Could you check a few things on this model? Use its own coordinates, in mm. Face numbers are marked on the shaded views. A direction names the side the tool comes from. Give positions to 0.01 mm unless a question says otherwise; leave off trailing zeros. Order: outer loops, then holes, each group sorted by start corner. A loop starts at its lowest first (then second) coordinate and runs counter-clockwise, first axis right, second up. Notation, with made-up numbers: (-25.75, -35) -> (-5.75, -35) arc R9 cw to (-5.75, -29) -> close; hole circle Ø7 at (21, 38.5). An arc over 180 degrees is marked (long way). Use one line per item in the form item = value. Start each with the question number.
from build123d import *

# Parameters (mm, degrees)
BOSS_EXTRUDE1_DEPTH = 4
CHAMFER1_SIZE       = 2


with BuildPart() as part:
    # Sketch2 → Boss-Extrude1 (new body)
    with BuildSketch(Plane(origin=(0, 0, 0), x_dir=(1, 0, 0), z_dir=(0, 1, 0))):
        Polygon((18, 8.5), (22.5, 8.5), (22.5, -8.5), (18, -8.5), (18, -13.5), (-18, -13.5), (-18, -8.5), (-22.5, -8.5), (-22.5, 8.5), (-18, 8.5), (-18, 13.5), (18, 13.5), align=None)
        Polygon((-8.5, -8.5), (8.5, -8.5), (0, -3), align=None, mode=Mode.SUBTRACT)
        Polygon((-4, 0), (-13, 6.5), (-13, 3.5), (-18, 3.5), (-18, -3.5), (-13, -3.5), (-13, -6.5), align=None, mode=Mode.SUBTRACT)
        Polygon((-8.5, 8.5), (0, 3), (8.5, 8.5), align=None, mode=Mode.SUBTRACT)
        Polygon((4, 0), (13, -6.5), (13, -3.5), (18, -3.5), (18, 3.5), (13, 3.5), (13, 6.5), align=None, mode=Mode.SUBTRACT)
    extrude(amount=BOSS_EXTRUDE1_DEPTH)

    # Chamfer1
    chamfer1_edges = [part.edges().sort_by_distance(p)[0] for p in [
        (22.5, 2, -8.5),
        (22.5, 2, 8.5),
        (18, 2, 13.5),
        (-18, 2, 13.5),
        (-22.5, 2, 8.5),
        (-22.5, 2, -8.5),
        (-18, 2, -13.5),
        (18, 2, -13.5),
    ]]
    chamfer(chamfer1_edges, length=CHAMFER1_SIZE)


solid = part.part
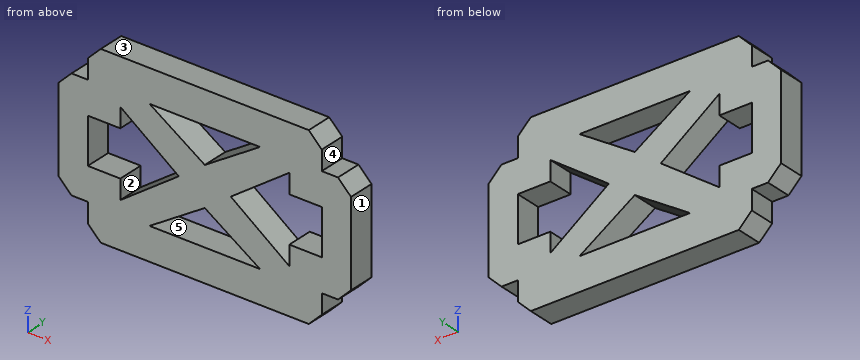
(1) Imagine slicing it at B-B (z = 4.75). Write out the boundary of the cut face in (x, y), plus the area to 3 significant figures.
(2) We'd pull the mould along X, two halves only. Please class the marked faces 3, 4 and 5: pulls with the +X half, pulls with the -X half, needs draft (parallel to the pull), parting line crosses it, or undercut.
(3) Which directions (+Z, -Z, +X, -X, +Y, -Y) give clear straight access to the entire face, cutting with the end or side of a thin tool? Please do the marked faces 1 and 2.
(4) I'm going to push flat-ended pins straight in: pin 1 Ø0.9 at (y, z) = (1.5, 9.5) entering from -X; pin 2 Ø1.2 at (x, y) = (18.5, 2) entering from +Z; pin 3 Ø0.8 at (x, y) = (-19, 1.5) entering from -Z. Where does each tip first touch, or does it pass through?
(5) Imagine slicing it at D-D (y = 3.15). Give the number of separate pieces and of enclosed holes in the cut face, plus the area to 4 significant figures.
(6) Please list where these lines run through material, in increasing order: probe 1 along Z at (x, y) = (-7.5, 3.55); probe 2 along Z at (x, y) = (-3.5, 2.65); probe 3 along X at (y, z) = (2.25, -1.5).
(7) Imagine slicing it at C-C (x = -2.5). Write out the boundary of the cut face in (y, z).
(8) Imagine slicing it at A-A (x = -17.5). Write out the boundary of the cut face in (y, z).
Calculated:
q1.outline = (-22.5, 0) -> (-13, 0) -> (-13, 4) -> (-22.5, 4) -> close; (-10.58, 0) -> (-2.7, 0) -> (-2.7, 4) -> (-10.58, 4) -> close; (2.7, 0) -> (10.58, 0) -> (10.58, 4) -> (2.7, 4) -> close; (13, 0) -> (22.5, 0) -> (22.5, 4) -> (13, 4) -> close
q1.area = 139 mm2
q2.face_3 = needs draft
q2.face_4 = pulls with the +X half
q2.face_5 = undercut
q3.face_1 = +Z, -Z, +X, +Y, -Y
q3.face_2 = +Y, -Y
q4.pin_1 = -18
q4.pin_2 = 11.6
q4.pin_3 = -8.5
q5.separate_pieces = 1
q5.enclosed_holes = 4
q5.area = 828.5 mm2
q6.probe_1 = -13.5 to -8.5, -7.85 to -2.53, 2.53 to 7.85, 8.5 to 13.5
q6.probe_2 = -13.5 to -8.5, -5.26 to 5.26, 8.5 to 13.5
q6.probe_3 = -22.5 to -18, -6.08 to 6.08, 18 to 22.5
q7.outline = (0, -13.5) -> (4, -13.5) -> (4, -8.5) -> (0, -8.5) -> close; (0, -4.62) -> (4, -4.62) -> (4, 4.62) -> (0, 4.62) -> close; (0, 8.5) -> (4, 8.5) -> (4, 13.5) -> (0, 13.5) -> close
q8.outline = (0, -12) -> (4, -12) -> (4, -3.5) -> (0, -3.5) -> close; (0, 3.5) -> (4, 3.5) -> (4, 12) -> (0, 12) -> close
